```python
from build123d import *

# Parameters (mm, degrees)
F1_DEPTH = 58
F2_W     = 36
F2_H     = 11
F3_DEPTH = 150
F5_DEPTH = 60


with BuildPart() as f1:
    # F0 (on Front) → F1 (new body)
    with BuildSketch(Plane.XZ):
        with BuildLine():
            Line((0, 9), (0, 0))
            Line((0, 0), (105, 0))
            Line((105, 0), (105, 9))
            Line((105, 9), (116, 9))
            ThreePointArc((116, 9), (107.506097, 29.506097), (87, 38))
            Line((87, 38), (18, 38))
            ThreePointArc((18, 38), (-2.506097, 29.506097), (-11, 9))
            Line((-11, 9), (0, 9))
        make_face()
    extrude(amount=-F1_DEPTH)

    # F2 (on Right) → F3 (cut, symmetric)
    with BuildSketch(Plane.YZ):
        with Locations((29, 32.5)):
            Rectangle(F2_W, F2_H)
    extrude(amount=F3_DEPTH, both=True, mode=Mode.SUBTRACT)

    # F4 (on face) → F5 (cut)
    with BuildSketch(Plane(origin=(0, 0, 0), x_dir=(1, 0, 0), z_dir=(0, 0, -1))):
        with BuildLine():
            Line((91, -22.5), (72, -22.5))
            ThreePointArc((72, -22.5), (65.5, -29), (72, -35.5))
            Line((72, -35.5), (91, -35.5))
            ThreePointArc((91, -35.5), (97.5, -29), (91, -22.5))
        make_face()
        with BuildLine():
            Line((33, -22.5), (14, -22.5))
            ThreePointArc((14, -22.5), (7.5, -29), (14, -35.5))
            Line((14, -35.5), (33, -35.5))
            ThreePointArc((33, -35.5), (39.5, -29), (33, -22.5))
        make_face()
    extrude(amount=-F5_DEPTH, mode=Mode.SUBTRACT)


solid = f1.part
```
Geometry: final body of the model. Coordinates: model frame, mm. A direction names the side the tool comes from. Round coordinates to 2 decimals unless told otherwise and drop trailing zeros. Loops run counter-clockwise (first coordinate to the right, second up) from the corner with the lowest first, then second, coordinate; pieces in that order, holes last. Notation, with made-up numbers: (30, -9.75) -> (78, -9.75) arc R13 ccw to (78, -2.75) -> close; hole circle Ø1 at (69.25, 55). An arc over 180 degrees is marked (long way). Write each question's results on one line, items separated by ' | '.
Item 1: Cut plane C-C on x = 64. Return the cut outline in (y, z).
Answers below:
outline: (0, 0) -> (58, 0) -> (58, 38) -> (47, 38) -> (47, 27) -> (11, 27) -> (11, 38) -> (0, 38) -> close
Item 2: Pin query (flat end, axial travel): pin 1 Ø5.5 at (x, y) = (-3.5, 38.5) entering from -Z; pin 2 Ø4 at (x, y) = (87.5, 24) entering from -Z; pin 3 Ø18 at (x, y) = (26, 28) entering from +Z; pin 4 Ø10 at (y, z) = (17.5, 26.5) entering from -X. Return the tip coordinate at first contact, or that it passes through.
Answers below:
pin 1: stops at z = 9 | pin 2: stops at z = 0 | pin 3: stops at z = 27 | pin 4: stops at x = -8.17
Item 3: Set-up query: faces 1 (the face through (0, 29, 5)), 2 (the face through (97.5, 29.1, 13.3)), 3 (the face through (53, 29, 27)). Return all of +Z, -Z, +X, -X, +Y, -Y with unobstructed straight access to the full face (end or side cutting, diameter ignored); none if empty.
Answers below:
face 1: -Z, -X, +Y, -Y | face 2: +Z, -Z | face 3: +Z, +X, -X
Item 4: Cut plane A-A on y = 31.5. Return the cut outline in (x, z), and give its area (3 significant figures).
Answers below:
outline: (-11, 9) -> (0, 9) -> (0, 0) -> (8, 0) -> (8, 27) -> (-4.74, 27) arc R29 ccw to start; (39, 0) -> (66, 0) -> (66, 27) -> (39, 27) -> close; (97, 0) -> (105, 0) -> (105, 9) -> (116, 9) arc R29 ccw to (109.74, 27) -> (97, 27) -> close | area: 1,490 mm²
Item 5: Cut plane B-B on z = 34. Return the cut outline in (x, y).
Answers below:
outline: (3.3, 0) -> (101.7, 0) -> (101.7, 11) -> (3.3, 11) -> close; (3.3, 47) -> (101.7, 47) -> (101.7, 58) -> (3.3, 58) -> close
Item 6: Line query: probe 1 along X at (y, z) = (29.5, 3); probe 2 along Y at (x, z) = (19.5, 12); probe 3 along X at (y, z) = (28.5, 24). Output: solid intervals per line, ascending. Write a range as [from, to].
Answers below:
probe 1: x = [0, 7.52], [39.48, 65.52], [97.48, 105] | probe 2: y = [0, 22.5], [35.5, 58] | probe 3: x = [-6.82, 7.52], [39.48, 65.52], [97.48, 111.82]
Item 7: Cut plane D-D on z = 14. Return the cut outline in (x, y), and give its area (3 significant figures).
Answers below:
outline: (-10.57, 0) -> (115.57, 0) -> (115.57, 58) -> (-10.57, 58) -> close; hole (14, 22.5) -> (33, 22.5) arc R6.5 ccw to (33, 35.5) -> (14, 35.5) arc R6.5 ccw to start; hole (72, 22.5) -> (91, 22.5) arc R6.5 ccw to (91, 35.5) -> (72, 35.5) arc R6.5 ccw to start | area: 6,560 mm²
Item 8: Pull-direction query (Y, two-part tool) for faces 4 (the face through (105, 29, 4)), 5 (the face through (52, 58, 19)), 6 (the face through (53, 47, 32)), 7 (the face through (81, 35.5, 13)); classes: pulls with the +Y half, pulls with the -Y half, needs draft (parallel to the pull), parting line crosses it, or undercut.
Answers below:
face 4: needs draft | face 5: pulls with the +Y half | face 6: undercut | face 7: undercut
